Design review of the part shown in the three views and the two pictorial views. Dimensions are in mm from the part's minimum x, y and z. A direction names the side the tool comes from. Round coordinates to 2 decimals unless told otherwise and drop trailing zeros. Loops run counter-clockwise (first coordinate to the right, second up) from the corner with the lowest first, then second, coordinate; pieces in that order, holes last. Notation, with made-up numbers: M 41.5,-3.75 L 74.5,-3.75 A18 ccw 74.5,18.25 Z; hole C 78.25,78 d11. An arc over 180 degrees is marked long. Return JSON: item names as keys, results as strings. Group by question number.
Q1. Consider section B-B (y = 16). State the section outline as (x, z) points, and give its area (3 significant figures).
Q2. Clearance check with flat-ended pins moving along their axes: pin 1 Ø1.5 at (y, z) = (25, 2) entering from +X; pin 2 Ø10 at (x, y) = (59, 39) entering from +Z; pin 3 Ø1.5 at (x, y) = (48.5, 33.5) entering from -Z; pin 4 Ø0.9 at (x, z) = (56.5, 8) entering from +Y. State where each tip first meets the part, or that it passes through.
Q3. Consider section A-A (x = 50.5). State the section outline as (y, z) points, and give its area (4 significant figures).
Q4. To check wall thickness, follow line 1 along Y through (x, z) = (58, 2.75); line 2 along Z through (x, y) = (17, 13.5); line 3 along X through (y, z) = (33, 0.5). State the ranges of each line that lie inside material, in increasing order.
Q5. Consider section D-D (z = 1.5). State the section outline as (x, y) points.
Q6. For the marked faces 1 and 2, list the 3-axis set-ups (+Z, -Z, +X, -X, +Y, -Y) from which the entire face can be reached by the end or side of a thin tool; tool diameter is ignored.
Q7. Consider section C-C (x = 68.5). State the section outline as (y, z) points, and give its area (3 significant figures).
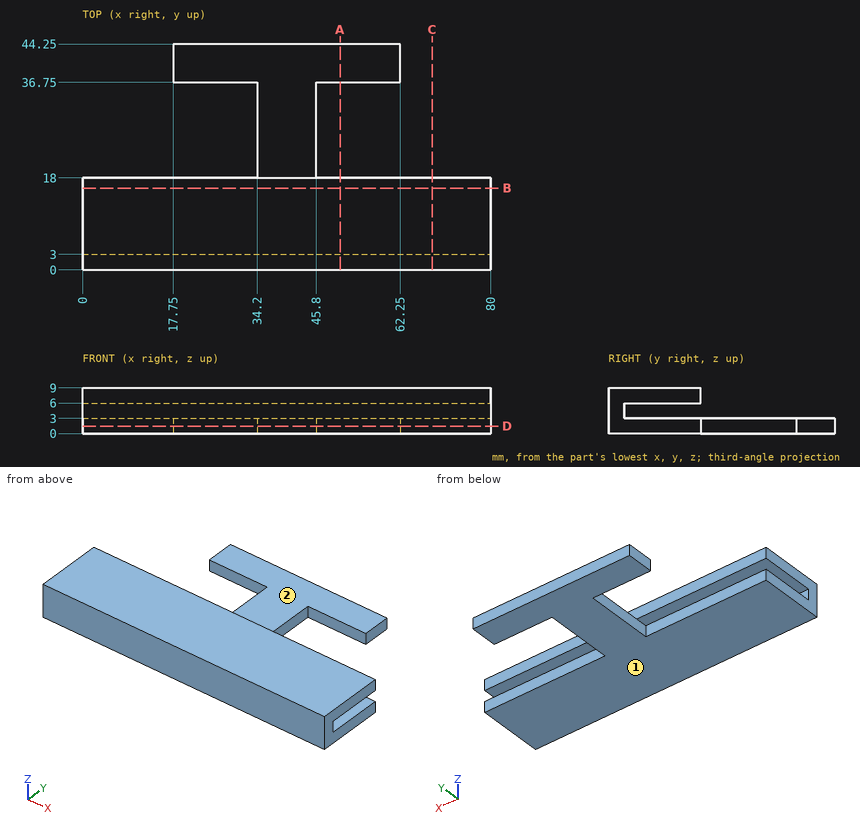
Values:
{
 "1": {"outline": "M 0,0 L 80,0 L 80,3 L 0,3 Z; M 0,6 L 80,6 L 80,9 L 0,9 Z", "area": "480 mm2"},
 "2": {"pin 1": "stops at x = 45.8", "pin 2": "stops at z = 3", "pin 3": "passes through", "pin 4": "stops at y = 18"},
 "3": {"outline": "M 0,0 L 18,0 L 18,3 L 3,3 L 3,6 L 18,6 L 18,9 L 0,9 Z; M 36.75,0 L 44.25,0 L 44.25,3 L 36.75,3 Z", "area": "139.5 mm2"},
 "4": {"line 1": "y = 0 to 18, 36.75 to 44.25", "line 2": "z = 0 to 3, 6 to 9", "line 3": "x = 34.2 to 45.8"},
 "5": {"outline": "M 0,0 L 80,0 L 80,18 L 45.8,18 L 45.8,36.75 L 62.25,36.75 L 62.25,44.25 L 17.75,44.25 L 17.75,36.75 L 34.2,36.75 L 34.2,18 L 0,18 Z"},
 "6": {"face 1": "-Z, +X, -X, +Y, -Y", "face 2": "+X, -X, +Y"},
 "7": {"outline": "M 0,0 L 18,0 L 18,3 L 3,3 L 3,6 L 18,6 L 18,9 L 0,9 Z", "area": "117 mm2"}
}
